```python
from build123d import *

# Parameters (mm, degrees)
F0_W     = 100
F0_H     = 100
F1_DEPTH = 80
F2_W     = 42.437702
F2_H     = 95
F2_W_2   = 50.062298
F2_H_2   = 54.196703
F2_H_3   = 38.303297
F3_DEPTH = 77.5
F5_DEPTH = 100


with BuildPart() as f1:
    # F0 (on Top) → F1 (new body)
    with BuildSketch(Plane.XY):
        with Locations((2.562298, 6.696703)):
            Rectangle(F0_W, F0_H)
    extrude(amount=F1_DEPTH)

    # F2 (on face) → F3 (cut)
    with BuildSketch(Plane.XY.offset(80)):
        with Locations((-23.718851, 6.696703)):
            Rectangle(F2_W, F2_H)
        with Locations((25.031149, 27.098351)):
            Rectangle(F2_W_2, F2_H_2)
        with Locations((25.031149, -21.651649)):
            Rectangle(F2_W_2, F2_H_3)
    extrude(amount=-F3_DEPTH, mode=Mode.SUBTRACT)

    # F4 (on face) → F5 (cut)
    with BuildSketch(Plane(origin=(-47.437702, 0, 0), x_dir=(0, -1, 0), z_dir=(-1, 0, 0))):
        Polygon((43.303297, 80), (-56.696703, 80), (43.303297, 47.50803), align=None)
    extrude(amount=-F5_DEPTH, mode=Mode.SUBTRACT)


solid = f1.part
```
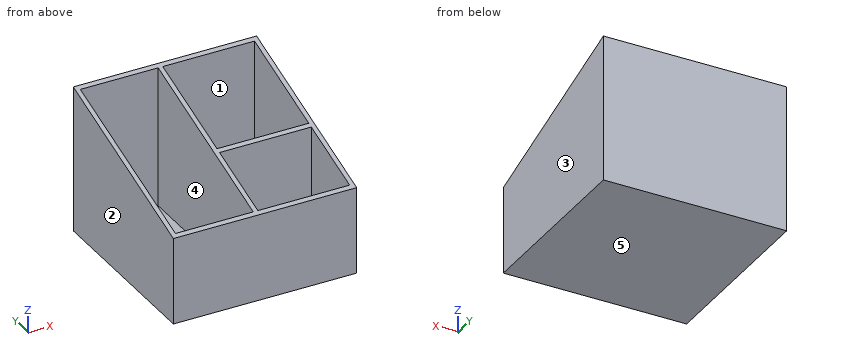
CAD build for the part. Positions are in the model's coordinates, mm. Face numbers are marked on the shaded views. A direction names the side the tool comes from. Round coordinates to 2 decimals unless told otherwise and drop trailing zeros. Write each loop counter-clockwise with the first axis right and the second up, starting at its lowest first coordinate (ties: lowest second). Pieces come first, ordered by that corner, then holes. Notation, with made-up numbers: M -12.5,45.25 L 44.5,45.25 A32 cw 44.5,84.25 Z; hole C 67.5,80.25 d10. An arc over 180 degrees is marked long. One line per question, with ' | ' between items.
1. Mould opens along X. For the marked faces 1, 2 and 3 say: pulls with the +X half, pulls with the -X half, needs draft (parallel to the pull), parting line crosses it, or undercut.
Working result:
face 1: undercut | face 2: pulls with the -X half | face 3: pulls with the +X half
2. Probe L1, parallel to X at y = 50, z = 16; L2, parallel to Y at x = 23, z = 32.5; L3, parallel to Y at x = -11, z = 16.5. List the from-to ranges inside material, lowest first. Write a range as from..to.
Working result:
L1: -47.44..-44.94, -2.5..0, 50.06..52.56 | L2: -43.3..-40.8, -2.5..0, 54.2..56.7 | L3: -43.3..-40.8, 54.2..56.7
3. Pin check, flat tips, straight feed: pin 1 Ø15 at (x, y) = (36, 39) entering from +Z; pin 2 Ø3 at (x, y) = (20.5, 10.5) entering from -Z. Stop position of each tip, or through.
Working result:
pin 1: z = 2.5 | pin 2: z = 0
4. Which spindle directions (+Z, -Z, +X, -X, +Y, -Y) get a long thin tool onto all of the face, cutting with end or side? Do the marked faces 4 and 5. Say none if no direction does.
Working result:
face 4: +Z | face 5: -Z, +X, -X, +Y, -Y
5. Cut at B-B on x = -19.5. Write the cut outline in (y, z).
Working result:
outline: M -43.3,0 L 56.7,0 L 56.7,80 L 54.2,79.19 L 54.2,2.5 L -40.8,2.5 L -40.8,48.32 L -43.3,47.51 Z
6. Cut at A-A on z = 20.5. Write the cut outline in (x, y), and give its area (3 significant figures).
Working result:
outline: M -47.44,-43.3 L 52.56,-43.3 L 52.56,56.7 L -47.44,56.7 Z; hole M -44.94,-40.8 L -2.5,-40.8 L -2.5,54.2 L -44.94,54.2 Z; hole M 0,-40.8 L 50.06,-40.8 L 50.06,-2.5 L 0,-2.5 Z; hole M 0,0 L 50.06,0 L 50.06,54.2 L 0,54.2 Z | area: 1,340 mm2
7. Cut at C-C on y = -32. Write the cut outline in (x, z), and give its area (3 significant figures).
Working result:
outline: M -47.44,0 L 52.56,0 L 52.56,51.18 L 50.06,51.18 L 50.06,2.5 L 0,2.5 L 0,51.18 L -2.5,51.18 L -2.5,2.5 L -44.94,2.5 L -44.94,51.18 L -47.44,51.18 Z | area: 615 mm2
8. Cut at D-D on z = 55. Write the cut outline in (x, y).
Working result:
outline: M -47.44,-20.25 L -44.94,-20.25 L -44.94,54.2 L -2.5,54.2 L -2.5,-20.25 L 0,-20.25 L 0,-2.5 L 50.06,-2.5 L 50.06,-20.25 L 52.56,-20.25 L 52.56,56.7 L -47.44,56.7 Z; hole M 0,0 L 50.06,0 L 50.06,54.2 L 0,54.2 Z
